```python
from build123d import *

# Parameters (mm, degrees)
SKETCH1_R                 = 12.7
BOSS_EXTRUDE1_DEPTH       = 6.35
BOSS_EXTRUDE6_START       = -6.35
BOSS_EXTRUDE6_DEPTH       = 6.35
SKETCH15_R                = 12.7
BOSS_EXTRUDE8_DEPTH       = 12.7
SKETCH17_R                = 1.651
CUT_EXTRUDE4_DEPTH        = 12.7
SKETCH18_R                = 3.81
CUT_EXTRUDE5_DEPTH        = 10.9027722
SKETCH19_R                = 8.255
CUT_EXTRUDE6_DEPTH        = 8.3627722
SKETCH20_R                = 9.525
CUT_EXTRUDE7_DEPTH        = 5.1877722
SKETCH21_R                = 1.2192
CUT_EXTRUDE8_DEPTH        = 4.3372278
SKETCH22_W                = 50.8
SKETCH22_H                = 50.8
BOSS_EXTRUDE9_DEPTH       = 6.35
F_6_CLEARANCE_HOLE1_D     = 3.7973
F_6_CLEARANCE_HOLE1_DEPTH = 25.4
F_6_CLEARANCE_HOLE1_TIP   = 1.140824014


with BuildPart() as part:
    # Sketch1 → Boss-Extrude1 (new body)
    with BuildSketch(Plane(origin=(0, 0, 0), x_dir=(1, 0, 0), z_dir=(0, 1, 0))):
        with Locations(Location((0, 0, 0), (0, 0, 270))):
            Circle(SKETCH1_R)
    extrude(amount=BOSS_EXTRUDE1_DEPTH)

    # Sketch14 → Boss-Extrude6 (add)
    with BuildSketch(Plane(origin=(0, 6.35, 0), x_dir=(1, 0, 0), z_dir=(0, 1, 0)).offset(BOSS_EXTRUDE6_START)):
        with BuildLine():
            Line((15.875, 12.7), (0, 12.7))
            ThreePointArc((0, 12.7), (8.980256121, 8.980256121), (12.7, 0))
            ThreePointArc((12.7, 0), (8.980256121, -8.980256121), (0, -12.7))
            Line((0, -12.7), (15.875, -12.7))
            Line((15.875, -12.7), (15.875, 12.7))
        make_face()
    extrude(amount=BOSS_EXTRUDE6_DEPTH)

    # Sketch15 → Boss-Extrude8 (add)
    with BuildSketch(Plane(origin=(15.875, 0, 0), x_dir=(0, 0, -1), z_dir=(1, 0, 0))):
        with Locations((0, 19.05)):
            Circle(SKETCH15_R)
        with BuildLine():
            ThreePointArc((-3e-08, 6.35), (-8.980256132, 10.06974389), (-12.7, 19.05))
            Line((-12.7, 19.05), (-12.7, 6.35))
            Line((-12.7, 6.35), (-3e-08, 6.35))
        make_face()
        with BuildLine():
            Line((12.7, 6.35), (12.7, 19.05))
            ThreePointArc((12.7, 19.05), (8.98025611, 10.069743868), (-3e-08, 6.35))
            Line((-3e-08, 6.35), (12.7, 6.35))
        make_face()
    extrude(amount=-BOSS_EXTRUDE8_DEPTH)

    # Sketch17 → Cut-Extrude4 (cut)
    with BuildSketch(Plane.ZY.offset(-3.175)):
        with Locations((0, 19.05)):
            Circle(SKETCH17_R)
    extrude(amount=-CUT_EXTRUDE4_DEPTH, mode=Mode.SUBTRACT)

    # Sketch18 → Cut-Extrude5 (cut)
    with BuildSketch(Plane.ZY.offset(-3.175)):
        with Locations((0, 19.05)):
            Circle(SKETCH18_R)
    extrude(amount=-CUT_EXTRUDE5_DEPTH, mode=Mode.SUBTRACT)

    # Sketch19 → Cut-Extrude6 (cut)
    with BuildSketch(Plane.ZY.offset(-3.175)):
        with Locations((0, 19.05)):
            Circle(SKETCH19_R)
    extrude(amount=-CUT_EXTRUDE6_DEPTH, mode=Mode.SUBTRACT)

    # Sketch20 → Cut-Extrude7 (cut)
    with BuildSketch(Plane.ZY.offset(-3.175)):
        with Locations((0, 19.05)):
            Circle(SKETCH20_R)
    extrude(amount=-CUT_EXTRUDE7_DEPTH, mode=Mode.SUBTRACT)

    # Sketch21 → Cut-Extrude8 (cut)
    with BuildSketch(Plane.ZY.offset(-11.5377722)):
        with Locations((5.4599967, 19.05)):
            Circle(SKETCH21_R)
        with Locations((-5.4599967, 19.05)):
            Circle(SKETCH21_R)
    extrude(amount=-CUT_EXTRUDE8_DEPTH, mode=Mode.SUBTRACT)

    # Sketch22 → Boss-Extrude9 (add)
    with BuildSketch(Plane.XZ):
        with Locations((1.5875, 0)):
            Rectangle(SKETCH22_W, SKETCH22_H)
    extrude(amount=BOSS_EXTRUDE9_DEPTH)

    # #6 Clearance Hole1
    with Locations(Plane(origin=(0, -6.35, 0), x_dir=(-1, 0, 0), z_dir=(0, -1, 0))):
        with Locations((-20.6375, 19.05), (17.4625, 19.05), (17.4625, -19.05), (-20.6375, -19.05)):
            Hole(F_6_CLEARANCE_HOLE1_D / 2, depth=F_6_CLEARANCE_HOLE1_DEPTH)
            with Locations((0, 0, -(F_6_CLEARANCE_HOLE1_DEPTH + F_6_CLEARANCE_HOLE1_TIP / 2))):  # 118° drill point
                Cone(0, F_6_CLEARANCE_HOLE1_D / 2, F_6_CLEARANCE_HOLE1_TIP, mode=Mode.SUBTRACT)


solid = part.part
```
Read the model definition and answer for the solid it produces. Units are mm, in the model's axes. A direction names the side the tool comes from. Give positions to 0.01 mm unless a question says otherwise; leave off trailing zeros. Write each loop counter-clockwise with the first axis right and the second up, starting at its lowest first coordinate (ties: lowest second). Pieces come first, ordered by that corner, then holes. Notation, with made-up numbers: (15.25, 66.5) -> (57.25, 66.5) arc R31 cw to (57.25, 101.5) -> close; hole circle Ø6 at (40.25, -1). An arc over 180 degrees is marked (long way). Answer as a JSON object with one key per item and string values.
1) Straight lines are drawn through the part: probe 1 along X at (y, z) = (-3.5, -19.05); probe 2 along Y at (x, z) = (9, 0) (3 decimals); probe 3 along Y at (x, z) = (5.5, 0) (3 decimals). For each, find the intervals that lie inside material, in ascending order. Write a range as from..to.
Findings below:
{"probe 1": "x = -23.81..-19.36, -15.56..18.74, 22.54..26.99", "probe 2": "y = -6.35..10.795, 27.305..31.75", "probe 3": "y = -6.35..9.525, 28.575..31.75"}
2) Section D-D on y = 13 is taken. Write down the section's boundary in (x, z) (3 decimals), then the cut area to 3 significant figures.
Findings below:
{"outline": "(3.175, -12.7) -> (15.875, -12.7) -> (15.875, 12.7) -> (3.175, 12.7) -> (3.175, 7.357) -> (8.363, 7.357) -> (8.363, 5.616) -> (11.538, 5.616) -> (11.538, -5.616) -> (8.363, -5.616) -> (8.363, -7.357) -> (3.175, -7.357) -> close", "area": "211 mm^2"}
3) Section A-A on z = -19.05 is taken. Write down the section's boundary in (x, y), then the cut area to 3 significant figures.
Findings below:
{"outline": "(-23.81, -6.35) -> (-19.36, -6.35) -> (-19.36, 0) -> (-23.81, 0) -> close; (-15.56, -6.35) -> (18.74, -6.35) -> (18.74, 0) -> (-15.56, 0) -> close; (22.54, -6.35) -> (26.99, -6.35) -> (26.99, 0) -> (22.54, 0) -> close", "area": "274 mm^2"}
4) For a pull along Y with two mould halves and no side action, classify faces 1 (the cylindrical face through (14.964, 17.585, 0.762)), 2 (the flat face through (1, -6.35, 0)), 3 (the flat face through (1, -3, -25.4)) as pulls with the +Y half, pulls with the -Y half, needs draft (parallel to the pull), parting line crosses it, or undercut.
Findings below:
{"face 1": "undercut", "face 2": "pulls with the -Y half", "face 3": "needs draft"}
5) Flat-ended cylindrical pins translate along their axes: pin 1 Ø3 at (x, y) = (11.5, 21.5) entering from +Z; pin 2 Ø10 at (x, y) = (10.5, 22) entering from -Z; pin 3 Ø8.5 at (y, z) = (21.5, 3.5) entering from -X. Find the tip coordinate at first contact, or state that the pin passes through.
Findings below:
{"pin 1": "stops at z = 12.66", "pin 2": "stops at z = -12.7", "pin 3": "stops at x = 8.36"}
6) A tool of negligible diameter and unlimited length cuts with its end or side. For faces 4 (the cylindrical face through (-12.697, 3.131, -0.279)), 5 (the flat face through (3.175, 10.8, -5.5)), 6 (the cylindrical face through (12.79, 22.828, -0.496)), from which of +Z, -Z, +X, -X, +Y, -Y can it reach the whole face along a straight path? Write none if from no direction.
Findings below:
{"face 4": "-X, +Y", "face 5": "+Z, -Z, -X, +Y", "face 6": "-X"}
7) Section C-C on x = 20 is taken. Write down the section's boundary in (y, z), then the cut area to 3 significant figures.
Findings below:
{"outline": "(-6.35, -25.4) -> (0, -25.4) -> (0, -20.84) -> (-6.35, -20.84) -> close; (-6.35, -17.26) -> (0, -17.26) -> (0, 17.26) -> (-6.35, 17.26) -> close; (-6.35, 20.84) -> (0, 20.84) -> (0, 25.4) -> (-6.35, 25.4) -> close", "area": "277 mm^2"}
